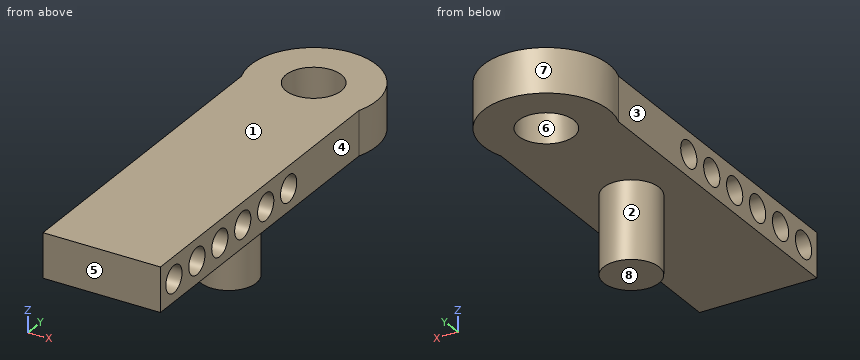
```python
from build123d import *

# Parameters (mm, degrees)
SKETCH2_R           = 10
BOSS_EXTRUDE2_DEPTH = 20
SKETCH8_R           = 6
CUT_EXTRUDE1_DEPTH  = 55.824018077
SKETCH6_R           = 6
CUT_EXTRUDE2_DEPTH  = 55.824018077
SKETCH9_R           = 12.5
CUT_EXTRUDE3_DEPTH  = 23
SKETCH11_R          = 12.5
BOSS_EXTRUDE4_DEPTH = 35


with BuildPart() as part:
    # Sketch2 → Boss-Extrude2 (new body)
    with BuildSketch(Plane.XY):
        with BuildLine():
            Line((-37.926977186, -74.415871925), (-37.926977186, -221.455871925))
            Line((-37.926977186, -221.455871925), (-90.926977186, -221.455871925))
            Line((-90.926977186, -221.455871925), (-90.926977186, -74.415871925))
            ThreePointArc((-90.926977186, -74.415871925), (-64.426977186, -36.091853848), (-37.926977186, -74.415871925))
        make_face()
        with Locations((-64.426977186, -64.415871925)):
            Circle(SKETCH2_R, mode=Mode.SUBTRACT)
    extrude(amount=BOSS_EXTRUDE2_DEPTH)

    # Sketch8 → Cut-Extrude1 (cut, through all)
    with BuildSketch(Plane.ZY.offset(90.926977186)):
        with Locations((10, -194.455871925)):
            Circle(SKETCH8_R)
        with Locations((10, -177.455871925)):
            Circle(SKETCH8_R)
        with Locations((10, -160.455871925)):
            Circle(SKETCH8_R)
        with Locations((10, -143.455871925)):
            Circle(SKETCH8_R)
        with Locations((10, -126.455871925)):
            Circle(SKETCH8_R)
    extrude(amount=-CUT_EXTRUDE1_DEPTH, mode=Mode.SUBTRACT)

    # Sketch6 → Cut-Extrude2 (cut, through all)
    with BuildSketch(Plane.ZY.offset(90.926977186)):
        with Locations((10, -211.455871925)):
            Circle(SKETCH6_R)
    extrude(amount=-CUT_EXTRUDE2_DEPTH, mode=Mode.SUBTRACT)

    # Sketch9 → Cut-Extrude3 (cut)
    with BuildSketch(Plane.XY.offset(20)):
        with Locations((-64.426977186, -64.415871925)):
            Circle(SKETCH9_R)
    extrude(amount=-CUT_EXTRUDE3_DEPTH, mode=Mode.SUBTRACT)

    # Sketch11 → Boss-Extrude4 (add)
    with BuildSketch(Plane.XY):
        with Locations((-64.426977186, -127.415871925)):
            Circle(SKETCH11_R)
    extrude(amount=-BOSS_EXTRUDE4_DEPTH)


solid = part.part
```
Input: part model. Units: mm. Frame: model coordinates. Face numbers are marked on the shaded views. A direction names the side the tool comes from. Coordinates: 2 decimals unless noted, no trailing zeros. Write each loop counter-clockwise with the first axis right and the second up, starting at its lowest first coordinate (ties: lowest second). Pieces come first, ordered by that corner, then holes. Notation, with made-up numbers: (45.5, 0.5) -> (102.5, 0.5) arc R36 cw to (102.5, 34.5) -> close; hole circle Ø5 at (18, 60.25). An arc over 180 degrees is marked (long way). Answer as a JSON object with one key per item and string values.
1. First-contact query: P1, Ø14, axis at y = -211.46, z = 10, coming from the -X side; P2, Ø14, axis at y = -177.46, z = 10, coming from the +X side; P3, Ø5, axis at x = -77, z = -25.5, coming from the -Y side. Flat tips, straight axial feed; report the tip coordinate or a pass-through.
Result set:
{"P1": "stops at x = -90.93", "P2": "stops at x = -37.93", "P3": "stops at y = -134.82"}
2. Material intervals for line 1 (Z direction, x = -72, y = -106); line 2 (Z direction, x = -85.5, y = -132); line 3 (X direction, y = -61.5, z = 2), sorted ascending. Write a range as from..to.
Result set:
{"line 1": "z = 0..20", "line 2": "z = 0..7.71, 12.29..20", "line 3": "x = -92.6..-76.58, -52.27..-36.25"}
3. Section A-A on x = -62.5. Return the cut outline in (y, z), then the cut area to 3 significant figures.
Result set:
{"outline": "(-221.46, 0) -> (-139.77, 0) -> (-139.77, -35) -> (-115.07, -35) -> (-115.07, 0) -> (-76.77, 0) -> (-76.77, 20) -> (-221.46, 20) -> close; (-52.07, 0) -> (-36.16, 0) -> (-36.16, 20) -> (-52.07, 20) -> close; hole circle Ø12 at (-211.46, 10); hole circle Ø12 at (-194.46, 10); hole circle Ø12 at (-177.46, 10); hole circle Ø12 at (-160.46, 10); hole circle Ø12 at (-143.46, 10); hole circle Ø12 at (-126.46, 10)", "area": "3,400 mm2"}
4. Mould query, pull axis Y, two halves, no side actions, for the marked faces 5, 6, 7 and 8. Classes: released by +Y, released by -Y, zero draft, split by the parting line, or undercut.
Result set:
{"face 5": "released by -Y", "face 6": "undercut", "face 7": "split by the parting line", "face 8": "zero draft"}
5. Access query for the marked faces 1, 2, 3 and 4. Directions: +Z, -Z, +X, -X, +Y, -Y. A direction counts if a zero-diameter tool reaches every point of the face in a straight line with its end or side. Return the directions, or none.
Result set:
{"face 1": "+Z, +X, -X, +Y, -Y", "face 2": "-Z", "face 3": "+Z, -Z, -X, -Y", "face 4": "+Z, -Z, +X, -Y"}
6. Section C-C on x = -80.5. Return the cut outline in (y, z), then the cut area to 3 significant figures.
Result set:
{"outline": "(-221.46, 0) -> (-41.09, 0) -> (-41.09, 20) -> (-221.46, 20) -> close; hole circle Ø12 at (-211.46, 10); hole circle Ø12 at (-194.46, 10); hole circle Ø12 at (-177.46, 10); hole circle Ø12 at (-160.46, 10); hole circle Ø12 at (-143.46, 10); hole circle Ø12 at (-126.46, 10)", "area": "2,930 mm2"}
7. Section D-D on y = -203. Return the cut outline in (x, z).
Result set:
{"outline": "(-90.93, 0) -> (-37.93, 0) -> (-37.93, 20) -> (-90.93, 20) -> close"}
8. Section B-B on z = 10. Count the separate pieces of the cut face and the enclosed holes in it, then the cut area to 3 significant figures.
Result set:
{"separate pieces": "7", "enclosed holes": "1", "area": "5,300 mm2"}
